from build123d import *

# Parameters (mm, degrees)
F0_W      = 127
F0_H      = 127
F1_DEPTH  = 127
F2_R      = 11.1125
F3_DEPTH  = 6.35
F4_R      = 11.1125
F6_DEPTH  = 6.35
F7_DEPTH  = 25.4
F5_R      = 11.1125
F8_DEPTH  = 6.35
F9_DEPTH  = 6.35
F10_R     = 11.1125
F11_DEPTH = 6.35
F13_R     = 11.1125
F14_DEPTH = 6.35
F12_R     = 11.1125
F15_DEPTH = 6.35


with BuildPart() as f1:
    # F0 (on Top) → F1 (new body)
    with BuildSketch(Plane.XY):
        with Locations((-24.36945, 11.884371)):
            Rectangle(F0_W, F0_H)
    extrude(amount=F1_DEPTH)

    # F2 (on face) → F3 (cut)
    with BuildSketch(Plane.XZ.offset(51.615629)):
        with Locations((-24.36945, 63.5)):
            Circle(F2_R)
    extrude(amount=-F3_DEPTH, mode=Mode.SUBTRACT)

    # F4 (on face) → F6 (cut)
    with BuildSketch(Plane(origin=(-87.86945, 0, 0), x_dir=(0, -1, 0), z_dir=(-1, 0, 0))):
        with Locations((29.390629, 104.775)):
            Circle(F4_R)
    extrude(amount=-F6_DEPTH, mode=Mode.SUBTRACT)

    # F4 (on face) → F7 (cut)
    with BuildSketch(Plane(origin=(-87.86945, 0, 0), x_dir=(0, -1, 0), z_dir=(-1, 0, 0))):
        with Locations((-11.884371, 63.5)):
            Circle(F4_R)
        with Locations((29.390629, 104.775)):
            Circle(F4_R)
        with Locations((-53.159371, 22.225)):
            Circle(F4_R)
    extrude(amount=-F7_DEPTH, mode=Mode.SUBTRACT)

    # F5 (on face) → F8 (cut)
    with BuildSketch(Plane.XY.offset(127)):
        with Locations((16.90555, -29.390629)):
            Circle(F5_R)
        with Locations((16.90555, 53.159371)):
            Circle(F5_R)
        with Locations((-65.64445, 53.159371)):
            Circle(F5_R)
        with Locations((-65.64445, -29.390629)):
            Circle(F5_R)
    extrude(amount=-F8_DEPTH, mode=Mode.SUBTRACT)

    # F5 (on face) → F9 (cut)
    with BuildSketch(Plane.XY.offset(127)):
        with Locations((-24.36945, 11.884371)):
            Circle(F5_R)
    extrude(amount=-F9_DEPTH, mode=Mode.SUBTRACT)

    # F10 (on face) → F11 (cut)
    with BuildSketch(Plane(origin=(0, 75.384371, 0), x_dir=(-1, 0, 0), z_dir=(0, 1, 0))):
        with Locations((-16.90555, 104.775)):
            Circle(F10_R)
        with Locations((-16.90555, 63.5)):
            Circle(F10_R)
        with Locations((-16.90555, 22.225)):
            Circle(F10_R)
        with Locations((65.64445, 22.225)):
            Circle(F10_R)
        with Locations((65.64445, 63.5)):
            Circle(F10_R)
        with Locations((65.64445, 104.775)):
            Circle(F10_R)
    extrude(amount=-F11_DEPTH, mode=Mode.SUBTRACT)

    # F13 (on face) → F14 (cut)
    with BuildSketch(Plane.YZ.offset(39.13055)):
        with Locations((53.159371, 104.775)):
            Circle(F13_R)
        with Locations((53.159371, 22.225)):
            Circle(F13_R)
        with Locations((-29.390629, 22.225)):
            Circle(F13_R)
        with Locations((-29.390629, 104.775)):
            Circle(F13_R)
    extrude(amount=-F14_DEPTH, mode=Mode.SUBTRACT)

    # F12 (on face) → F15 (cut)
    with BuildSketch(Plane(origin=(0, 0, 0), x_dir=(1, 0, 0), z_dir=(0, 0, -1))):
        with Locations((-65.64445, -53.159371)):
            Circle(F12_R)
        with Locations((16.90555, 29.390629)):
            Circle(F12_R)
    extrude(amount=-F15_DEPTH, mode=Mode.SUBTRACT)


solid = f1.part
Verification items for the finished model (mm, model axes). A direction names the side the tool comes from. Round coordinates to 2 decimals unless told otherwise and drop trailing zeros. Loops run counter-clockwise (first coordinate to the right, second up) from the corner with the lowest first, then second, coordinate; pieces in that order, holes last. Notation, with made-up numbers: (83.25, 49) - (142.25, 49) arc R12 cw to (142.25, 60) - close; hole circle Ø1 at (66.25, -37). An arc over 180 degrees is marked (long way). Use a Markdown table: item, result. Add a question column.
1. Access from +Z, -Z, +X, -X, +Y, -Y to the whole of each face (thin tool, end or side, straight path). Record for faces 5 (the face through (36, -30.837, 115.793)), 6 (the face through (-32.56, -48.49, 71.01)), 7 (the face through (-75.35, -35.36, 114.15)), 8 (the face through (-33.188, 5.123, 123.869)), 9 (the face through (-71.62, 72.25, 72.87)).
2. Thickness scan on probe 1 along X at (y, z) = (71, 63); probe 2 along X at (y, z) = (70, 28); probe 3 along Z at (x, y) = (34, -28). Record the ranges inside material, lowest first. Write a range as [from, to].
3. Section check B-B, the plane z = 112. Record the boundary of the cut face in (x, y), plus the area to 3 significant figures.
4. Section check C-C, the plane y = -35. Record the boundary of the cut face in (x, z).
5. Section check A-A, the plane y = 3. Record the boundary of the cut face in (x, z) (3 decimals).
6. Release check for a two-part mould opening along X. For faces 1 (the face through (-66, 53, 6.35)), 2 (the face through (-75.35, 13.33, 74.52)), 3 (the face through (32.781, -30, 105)), 4 (the face through (-65, 69.034, 22)) record: released by +X, released by -X, zero draft, split by the parting line, or undercut.
7. Gauge pin test, flat ends, axial feed: pin 1 (20 mm diameter, centred on y = 11.88, z = 63.5, fed in from -X); pin 2 (20 mm diameter, centred on x = 16.91, y = -29.39, fed in from +Z); pin 3 (18 mm diameter, centred on y = 51.5, z = 20.5, fed in from -X); pin 4 (18 mm diameter, centred on x = 18, z = 63.5, fed in from +Y). Record the tip position at first contact, or that the pin passes through.
Checks:
| question | item | result |
|---|---|---|
| 1 | face 5 | +X |
| 1 | face 6 | -Y |
| 1 | face 7 | -X |
| 1 | face 8 | +Z |
| 1 | face 9 | +Y |
| 2 | probe 1 | x = [-87.87, -76.75], [-54.54, 5.8], [28.01, 39.13] |
| 2 | probe 2 | x = [-87.87, -75.14], [-56.15, 7.41], [26.4, 39.13] |
| 2 | probe 3 | z = [0, 11.2], [33.25, 93.75], [115.8, 127] |
| 3 | outline | (-87.87, -51.62) - (39.13, -51.62) - (39.13, -37.83) - (32.78, -37.83) - (32.78, -20.95) - (39.13, -20.95) - (39.13, 44.72) - (32.78, 44.72) - (32.78, 61.6) - (39.13, 61.6) - (39.13, 75.38) - (25.35, 75.38) - (25.35, 69.03) - (8.46, 69.03) - (8.46, 75.38) - (-57.2, 75.38) - (-57.2, 69.03) - (-74.09, 69.03) - (-74.09, 75.38) - (-87.87, 75.38) - (-87.87, -20.95) - (-62.47, -20.95) - (-62.47, -37.83) - (-87.87, -37.83) - close |
| 3 | area | 15,300 mm^2 |
| 4 | outline | (-87.87, 0) - (7.31, 0) - (7.31, 6.35) - (26.5, 6.35) - (26.5, 0) - (39.13, 0) - (39.13, 12.63) - (32.78, 12.63) - (32.78, 31.82) - (39.13, 31.82) - (39.13, 95.18) - (32.78, 95.18) - (32.78, 114.37) - (39.13, 114.37) - (39.13, 127) - (26.5, 127) - (26.5, 120.65) - (7.31, 120.65) - (7.31, 127) - (-56.05, 127) - (-56.05, 120.65) - (-75.24, 120.65) - (-75.24, 127) - (-87.87, 127) - (-87.87, 114.37) - (-62.47, 114.37) - (-62.47, 95.18) - (-87.87, 95.18) - close |
| 5 | outline | (-87.869, 0) - (39.131, 0) - (39.131, 127) - (-17.694, 127) - (-17.694, 120.65) - (-31.044, 120.65) - (-31.044, 127) - (-87.869, 127) - (-87.869, 70.175) - (-62.469, 70.175) - (-62.469, 56.825) - (-87.869, 56.825) - close |
| 6 | face 1 | undercut |
| 6 | face 2 | zero draft |
| 6 | face 3 | released by +X |
| 6 | face 4 | undercut |
| 7 | pin 1 | stops at x = -62.47 |
| 7 | pin 2 | stops at z = 120.65 |
| 7 | pin 3 | stops at x = -87.87 |
| 7 | pin 4 | stops at y = 69.03 |
